```python
from build123d import *

# Parameters (mm, degrees)
F0_R     = 25
F0_R_2   = 15
F1_DEPTH = 1.5
F2_R     = 16.5
F2_R_2   = 15.25
F3_DEPTH = 27
F4_R     = 2


with BuildPart() as f1:
    # F0 (on Front) → F1 (new body)
    with BuildSketch(Plane.XZ):
        Circle(F0_R)
        Circle(F0_R_2, mode=Mode.SUBTRACT)
    extrude(amount=F1_DEPTH)

    # F2 (on Front) → F3 (join)
    with BuildSketch(Plane.XZ):
        Circle(F2_R)
        Circle(F2_R_2, mode=Mode.SUBTRACT)
    extrude(amount=F3_DEPTH)

    # F4
    f4_edges = [f1.edges().sort_by_distance(p)[0] for p in [
        (-16.5, -1.5, 0),
    ]]
    fillet(f4_edges, radius=F4_R)


solid = f1.part
```
Input: part model. Units: mm. Frame: model coordinates. A direction names the side the tool comes from. Give positions to 0.01 mm unless a question says otherwise; leave off trailing zeros. Order: outer loops, then holes, each group sorted by start corner. A loop starts at its lowest first (then second) coordinate and runs counter-clockwise, first axis right, second up. Notation, with made-up numbers: M 45.25,12.5 L 64.25,12.5 A21 ccw 64.25,36.5 Z; hole C 35,68 d11. An arc over 180 degrees is marked long. One line per question, with ' | ' between items. Start each with the question number.
1. Section query C-C (y = -18.5). Return the cut outline in (x, z).
2. Section query D-D (z = -20.5). Return the cut outline in (x, y), and give its area (3 significant figures).
3. Material intervals for probe 1 along Z at (x, y) = (0, -0.3); probe 2 along Z at (x, y) = (0, -6.25), sorted ascending. Write a range as [from, to].
4. First-contact query: pin 1 Ø1.5 at (x, y) = (8.5, -8.5) entering from +Z; pin 2 Ø1 at (x, y) = (14, -16) entering from +Z; pin 3 Ø5 at (x, y) = (-16.5, -23) entering from +Z. Flat tips, straight axial feed; report the tip coordinate or a pass-through.
5. Access query for faces 5 (the face through (0, -1.5, 19)), 6 (the face through (11, 0, -11)). Directions: +Z, -Z, +X, -X, +Y, -Y. A direction counts if a zero-diameter tool reaches every point of the face in a straight line with its end or side. Return the directions, or none.
6. Section query A-A (z = 0). Return the cut outline in (x, y), and give its area (3 significant figures).
7. Pull-direction query (Z, two-part tool) for faces 1 (the face through (-14.985, -0.74, 0.66)), 2 (the face through (23.846, -0.74, 7.509)), 3 (the face through (-12.1, -14.07, -9.28)), 4 (the face through (15, -27, -5)); classes: released by +Z, released by -Z, zero draft, split by the parting line, or undercut.
8. Section query B-B (x = 0). Return the cut outline in (y, z), and give its area (3 significant figures).
Here are the results:
1) outline: C 0,0 d33; hole C 0,0 d30.5
2) outline: M -14.31,-1.5 L 14.31,-1.5 L 14.31,0 L -14.31,0 Z | area: 42.9 mm²
3) probe 1: [-25, -15], [15, 25] | probe 2: [-16.5, -15.25], [15.25, 16.5]
4) pin 1: z = 14.57 | pin 2: z = 9.49 | pin 3: z = 8.73
5) face 5: -Y | face 6: +Z, -Z, +X, -X, +Y
6) outline: M -25,-1.5 L -18.5,-1.5 A2 cw -16.5,-3.5 L -16.5,-27 L -15.25,-27 L -15.25,-1.5 L -15,-1.5 L -15,0 L -25,0 Z; M 15,-1.5 L 15.25,-1.5 L 15.25,-27 L 16.5,-27 L 16.5,-3.5 A2 cw 18.5,-1.5 L 25,-1.5 L 25,0 L 15,0 Z | area: 95.5 mm²
7) face 1: undercut | face 2: split by the parting line | face 3: undercut | face 4: zero draft
8) outline: M -27,-16.5 L -3.5,-16.5 A2 cw -1.5,-18.5 L -1.5,-25 L 0,-25 L 0,-15 L -1.5,-15 L -1.5,-15.25 L -27,-15.25 Z; M -27,15.25 L -1.5,15.25 L -1.5,15 L 0,15 L 0,25 L -1.5,25 L -1.5,18.5 A2 cw -3.5,16.5 L -27,16.5 Z | area: 95.5 mm²
